The model under review builds one solid part; all positions refer to its coordinate system, in mm. A direction names the side the tool comes from. Give positions to 0.01 mm unless a question says otherwise; leave off trailing zeros. Order: outer loops, then holes, each group sorted by start corner. A loop starts at its lowest first (then second) coordinate and runs counter-clockwise, first axis right, second up. Notation, with made-up numbers: (28.5, 5) - (74.5, 5) arc R28 ccw to (74.5, 23) - close; hole circle Ø9 at (-21.75, 5.25). An arc over 180 degrees is marked (long way). Use a Markdown table: item, result. Add a question column.
```python
from build123d import *

# Parameters (mm, degrees)
SALIENTE_EXTRUIR1_DEPTH      = 30
SALIENTE_EXTRUIR1_DEPTH_BACK = 30
CHAFL_N1_SIZE                = 5
CHAFL_N2_SIZE                = 5
CROQUIS2_R                   = 6.5
CORTAR_EXTRUIR1_DEPTH        = 9
CORTAR_EXTRUIR2_REACH        = 175.45
CROQUIS3_R                   = 4.25
CROQUIS4_R                   = 4
CORTAR_EXTRUIR3_DEPTH        = 30


with BuildPart() as part:
    # Croquis1 → Saliente-Extruir1 (new, two sides: drawn at the far end of the back side and taken through both)
    with BuildSketch(Plane(origin=(0, 0, 0), x_dir=(0, 0, -1), z_dir=(1, 0, 0)).offset(-SALIENTE_EXTRUIR1_DEPTH_BACK)):
        Polygon((0, 0), (-40, 0), (-40, -72), (-38, -72), (-38, -168), (0, -168), align=None)
    extrude(amount=SALIENTE_EXTRUIR1_DEPTH + SALIENTE_EXTRUIR1_DEPTH_BACK)

    # Chafl_n1
    chafl_n1_edges = [part.edges().sort_by_distance(p)[0] for p in [
        (0, 0, 0),
    ]]
    chamfer(chafl_n1_edges, length=CHAFL_N1_SIZE)

    # Chafl_n2
    chafl_n2_edges = [part.edges().sort_by_distance(p)[0] for p in [
        (30, 0, 22.5),
        (-30, 0, 22.5),
    ]]
    chamfer(chafl_n2_edges, length=CHAFL_N2_SIZE)

    # Croquis2 → Cortar-Extruir1 (cut)
    with BuildSketch(Plane(origin=(0, 0, 0), x_dir=(-1, 0, 0), z_dir=(0, 0, -1))):
        with Locations((-20, -12)):
            Circle(CROQUIS2_R)
        with Locations((20, -12)):
            Circle(CROQUIS2_R)
        with Locations((-20, -60)):
            Circle(CROQUIS2_R)
        with Locations((20, -60)):
            Circle(CROQUIS2_R)
    extrude(amount=-CORTAR_EXTRUIR1_DEPTH, mode=Mode.SUBTRACT)

    # Croquis3 → Cortar-Extruir2 (cut, up to next)
    with BuildSketch(Plane(origin=(0, 0, 9), x_dir=(-1, 0, 0), z_dir=(0, 0, -1)), mode=Mode.PRIVATE) as cortar_extruir2_sk1:
        with Locations((-20, -12)):
            Circle(CROQUIS3_R)
    cortar_extruir2_tool1 = extrude(cortar_extruir2_sk1.sketch, amount=-CORTAR_EXTRUIR2_REACH, mode=Mode.PRIVATE) & part.part
    # Croquis3 → Cortar-Extruir2 (cut, up to next)
    with BuildSketch(Plane(origin=(0, 0, 9), x_dir=(-1, 0, 0), z_dir=(0, 0, -1)), mode=Mode.PRIVATE) as cortar_extruir2_sk2:
        with Locations((20, -12)):
            Circle(CROQUIS3_R)
    cortar_extruir2_tool2 = extrude(cortar_extruir2_sk2.sketch, amount=-CORTAR_EXTRUIR2_REACH, mode=Mode.PRIVATE) & part.part
    # Croquis3 → Cortar-Extruir2 (cut, up to next)
    with BuildSketch(Plane(origin=(0, 0, 9), x_dir=(-1, 0, 0), z_dir=(0, 0, -1)), mode=Mode.PRIVATE) as cortar_extruir2_sk3:
        with Locations((20, -60)):
            Circle(CROQUIS3_R)
    cortar_extruir2_tool3 = extrude(cortar_extruir2_sk3.sketch, amount=-CORTAR_EXTRUIR2_REACH, mode=Mode.PRIVATE) & part.part
    # Croquis3 → Cortar-Extruir2 (cut, up to next)
    with BuildSketch(Plane(origin=(0, 0, 9), x_dir=(-1, 0, 0), z_dir=(0, 0, -1)), mode=Mode.PRIVATE) as cortar_extruir2_sk4:
        with Locations((-20, -60)):
            Circle(CROQUIS3_R)
    cortar_extruir2_tool4 = extrude(cortar_extruir2_sk4.sketch, amount=-CORTAR_EXTRUIR2_REACH, mode=Mode.PRIVATE) & part.part
    add(cortar_extruir2_tool1.solids().sort_by_distance((20, -12, 9))[0], mode=Mode.SUBTRACT)
    add(cortar_extruir2_tool2.solids().sort_by_distance((-20, -12, 9))[0], mode=Mode.SUBTRACT)
    add(cortar_extruir2_tool3.solids().sort_by_distance((-20, -60, 9))[0], mode=Mode.SUBTRACT)
    add(cortar_extruir2_tool4.solids().sort_by_distance((20, -60, 9))[0], mode=Mode.SUBTRACT)

    # Croquis4 → Cortar-Extruir3 (cut)
    with BuildSketch(Plane.XZ.offset(168)):
        with Locations(Location((-22, 30, 0), (0, 0, 270))):
            Circle(CROQUIS4_R)
        with Locations(Location((-22, 8, 0), (0, 0, 270))):
            Circle(CROQUIS4_R)
        with Locations(Location((22, 30, 0), (0, 0, 270))):
            Circle(CROQUIS4_R)
        with Locations(Location((22, 8, 0), (0, 0, 270))):
            Circle(CROQUIS4_R)
    extrude(amount=-CORTAR_EXTRUIR3_DEPTH, mode=Mode.SUBTRACT)


solid = part.part
```
Q1. We need section C-C (y = -12). Write out the cut boundary in (x, z), plus the area to 3 significant figures.
Q2. We need section B-B (y = -148). Write out the cut boundary in (x, z), plus the area to 3 significant figures.
Q3. Wall thickness on probe 1 along Y at (x, z) = (20, 31); probe 2 along X at (y, z) = (-149.5, 30); probe 3 along Y at (x, z) = (20, 23): over which ranges is each line inside the solid? List them lowest first.
Q4. Clearance check with flat-ended pins moving along their axes: P1, Ø15, axis at x = 20, y = -60, coming from the +Z side; P2, Ø6.5, axis at x = -22.5, y = -14, coming from the -Z side; P3, Ø1.5, axis at x = -15.5, y = -81.5, coming from the +Z side; P4, Ø4, axis at x = -23, z = 8.5, coming from the -Y side. State where each tip first meets the part, or that it passes through.
Q5. Machinability: for faces 1 (the flat face through (0, -168, 19)), 2 (the cylindrical face through (26.494, -11.714, 4.437)), 3 (the flat face through (-22, -138, 8)), which of the approach directions +Z, -Z, +X, -X, +Y, -Y give a long, thin tool a straight path to every point of the face, cutting with its end or side? Answer none if there is none.
Q6. We need section D-D (x = 22). Count the separate pieces of the cut face and the enclosed holes in it, plus the area to 3 significant figures.
Q7. Draft analysis for pull direction Z (two halves, no side actions). For faces 4 (the flat face through (-24.2, -61.4, 9)), 5 (the flat face through (22, -138, 30)), 6 (the flat face through (-30, -85, 20)), state which applies: pulls with the +Z half, pulls with the -Z half, needs draft (parallel to the pull), parting line crosses it, or undercut.
Q8. We need section A-A (z = 35.5). Write out the cut boundary in (x, y), plus the area to 3 significant figures.
Here are the results:
| question | item | result |
|---|---|---|
| 1 | outline | (-30, 0) - (-26.5, 0) - (-26.5, 9) - (-24.25, 9) - (-24.25, 40) - (-30, 40) - close; (-15.75, 9) - (-13.5, 9) - (-13.5, 0) - (13.5, 0) - (13.5, 9) - (15.75, 9) - (15.75, 40) - (-15.75, 40) - close; (24.25, 9) - (26.5, 9) - (26.5, 0) - (30, 0) - (30, 40) - (24.25, 40) - close |
| 1 | area | 1,640 mm2 |
| 2 | outline | (-30, 0) - (30, 0) - (30, 38) - (-30, 38) - close; hole circle Ø8 at (-22, 8); hole circle Ø8 at (-22, 30); hole circle Ø8 at (22, 8); hole circle Ø8 at (22, 30) |
| 2 | area | 2,080 mm2 |
| 3 | probe 1 | -138 to -64.25, -55.75 to -16.25, -7.75 to 0 |
| 3 | probe 2 | -30 to -26, -18 to 18, 26 to 30 |
| 3 | probe 3 | -168 to -64.25, -55.75 to -16.25, -7.75 to 0 |
| 4 | P1 | z = 40 |
| 4 | P2 | z = 9 |
| 4 | P3 | z = 38 |
| 4 | P4 | y = -138 |
| 5 | face 1 | +Z, -Z, +X, -X, -Y |
| 5 | face 2 | -Z |
| 5 | face 3 | -Y |
| 6 | separate pieces | 3 |
| 6 | enclosed holes | 0 |
| 6 | area | 5,350 mm2 |
| 7 | face 4 | pulls with the -Z half |
| 7 | face 5 | undercut |
| 7 | face 6 | needs draft |
| 8 | outline | (-30, -168) - (30, -168) - (30, -5) - (25, 0) - (-25, 0) - (-30, -5) - close; hole circle Ø8.5 at (-20, -60); hole circle Ø8.5 at (-20, -12); hole circle Ø8.5 at (20, -60); hole circle Ø8.5 at (20, -12) |
| 8 | area | 9,830 mm2 |
